```python
from build123d import *

# Parameters (mm, degrees)
BASPROSKE_W        = 12.7
BASPROSKE_H        = 33
TOOTHCUT_DEPTH     = 49.366207211
TEETHCUTS_COUNT    = 20
TEETHCUTS_ANGLE    = 342
BORSKE_R           = 5
BORE_DEPTH         = 50.0000508
CUT_EXTRUDE1_START = -6.35
CUT_EXTRUDE1_DEPTH = 6.35


with BuildPart() as part:
    # BasProSke → Base-Revolve (revolve)
    with BuildSketch(Plane(origin=(0, 0, 0), x_dir=(1, 0, 0), z_dir=(0, 1, 0)), mode=Mode.PRIVATE) as base_revolve_sk:
        with Locations((6.35, 16.5)):
            Rectangle(BASPROSKE_W, BASPROSKE_H)
    revolve(base_revolve_sk.sketch.rotate(Axis((-10, 0, 0), (1, 0, 0)), 180), axis=Axis((-10, 0, 0), (1, 0, 0)))

    # TooCutSke → ToothCut (cut, through all)
    with BuildSketch(Plane(origin=(0, 0, 0), x_dir=(0, 0, -1), z_dir=(1, 0, 0))):
        with BuildLine():
            ThreePointArc((1.489278925, 26.206717637), (0, 26.249), (-1.489278925, 26.206717637))
            ThreePointArc((-1.489278925, 26.206717637), (-2.448651415, 29.690511169), (-4.401620335, 32.730762038))
            ThreePointArc((-4.401620335, 32.730762038), (0, 33.0254), (4.401620335, 32.730762038))
            ThreePointArc((4.401620335, 32.730762038), (2.448651415, 29.690511169), (1.489278925, 26.206717637))
        make_face()
    toothcut = extrude(amount=TOOTHCUT_DEPTH, mode=Mode.SUBTRACT)

    # TeethCuts: ToothCut ×20 about axis
    teethcuts_axis = Axis((-10, 0, 0), (1, 0, 0))
    for i in range(1, TEETHCUTS_COUNT):
        add(toothcut.rotate(teethcuts_axis, i * TEETHCUTS_ANGLE / (TEETHCUTS_COUNT - 1)), mode=Mode.SUBTRACT)

    # BorSke → Bore (cut, symmetric)
    with BuildSketch(Plane(origin=(0, 0, 0), x_dir=(0, 0, -1), z_dir=(1, 0, 0))):
        with Locations(Location((0, 0, 0), (0, 0, 180))):
            Circle(BORSKE_R)
    extrude(amount=BORE_DEPTH, both=True, mode=Mode.SUBTRACT)

    # Sketch1 → Cut-Extrude1 (cut)
    with BuildSketch(Plane(origin=(12.7, 0, 0), x_dir=(0, 0, -1), z_dir=(1, 0, 0)).offset(CUT_EXTRUDE1_START)):
        with BuildLine():
            ThreePointArc((-32.707837592, 4.381479207), (-29.676574647, 2.442440757), (-26.206717637, 1.489278925))
            ThreePointArc((-26.206717637, 1.489278925), (-26.249, 0), (-26.206717637, -1.489278925))
            ThreePointArc((-26.206717637, -1.489278925), (-29.676574647, -2.442440757), (-32.707837592, -4.381479207))
            ThreePointArc((-32.707837592, -4.381479207), (-32.59371524, -5.162337346), (-32.460953611, -5.940243315))
            ThreePointArc((-32.460953611, -5.940243315), (-28.978855401, -6.847666703), (-25.384282076, -6.68193269))
            ThreePointArc((-25.384282076, -6.68193269), (-24.964282496, -8.111387085), (-24.463857082, -9.514709543))
            ThreePointArc((-24.463857082, -9.514709543), (-27.469343998, -11.493465099), (-29.753050541, -14.274312016))
            ThreePointArc((-29.753050541, -14.274312016), (-29.403215298, -14.981686491), (-29.036565322, -15.680493433))
            ThreePointArc((-29.036565322, -15.680493433), (-25.444483881, -15.467476836), (-22.077056123, -14.199070178))
            ThreePointArc((-22.077056123, -14.199070178), (-21.235887085, -15.428775087), (-20.326303746, -16.608774097))
            ThreePointArc((-20.326303746, -16.608774097), (-22.573222567, -19.419428996), (-23.885827601, -22.76987571))
            ThreePointArc((-23.885827601, -22.76987571), (-23.334523779, -23.334523779), (-22.76987571, -23.885827601))
            ThreePointArc((-22.76987571, -23.885827601), (-19.419428996, -22.573222567), (-16.608774097, -20.326303746))
            ThreePointArc((-16.608774097, -20.326303746), (-15.428775087, -21.235887085), (-14.199070178, -22.077056123))
            ThreePointArc((-14.199070178, -22.077056123), (-15.467476836, -25.444483881), (-15.680493433, -29.036565322))
            ThreePointArc((-15.680493433, -29.036565322), (-14.981686491, -29.403215298), (-14.274312016, -29.753050541))
            ThreePointArc((-14.274312016, -29.753050541), (-11.493465099, -27.469343998), (-9.514709543, -24.463857082))
            ThreePointArc((-9.514709543, -24.463857082), (-8.111387085, -24.964282496), (-6.68193269, -25.384282076))
            ThreePointArc((-6.68193269, -25.384282076), (-6.847666703, -28.978855401), (-5.940243315, -32.460953611))
            ThreePointArc((-5.940243315, -32.460953611), (-5.162337346, -32.59371524), (-4.381479207, -32.707837592))
            ThreePointArc((-4.381479207, -32.707837592), (-2.442440757, -29.676574647), (-1.489278925, -26.206717637))
            ThreePointArc((-1.489278925, -26.206717637), (0, -26.249), (1.489278925, -26.206717637))
            ThreePointArc((1.489278925, -26.206717637), (2.442440757, -29.676574647), (4.381479207, -32.707837592))
            ThreePointArc((4.381479207, -32.707837592), (5.162337346, -32.59371524), (5.940243315, -32.460953611))
            ThreePointArc((5.940243315, -32.460953611), (6.847666703, -28.978855401), (6.68193269, -25.384282076))
            ThreePointArc((6.68193269, -25.384282076), (8.111387085, -24.964282496), (9.514709543, -24.463857082))
            ThreePointArc((9.514709543, -24.463857082), (11.493465099, -27.469343998), (14.274312016, -29.753050541))
            ThreePointArc((14.274312016, -29.753050541), (14.981686491, -29.403215298), (15.680493433, -29.036565322))
            ThreePointArc((15.680493433, -29.036565322), (15.467476836, -25.444483881), (14.199070178, -22.077056123))
            ThreePointArc((14.199070178, -22.077056123), (15.428775087, -21.235887085), (16.608774097, -20.326303746))
            ThreePointArc((16.608774097, -20.326303746), (19.419428996, -22.573222567), (22.76987571, -23.885827601))
            ThreePointArc((22.76987571, -23.885827601), (23.334523779, -23.334523779), (23.885827601, -22.76987571))
            ThreePointArc((23.885827601, -22.76987571), (22.573222567, -19.419428996), (20.326303746, -16.608774097))
            ThreePointArc((20.326303746, -16.608774097), (21.235887085, -15.428775087), (22.077056123, -14.199070178))
            ThreePointArc((22.077056123, -14.199070178), (25.444483881, -15.467476836), (29.036565322, -15.680493433))
            ThreePointArc((29.036565322, -15.680493433), (29.403215298, -14.981686491), (29.753050541, -14.274312016))
            ThreePointArc((29.753050541, -14.274312016), (27.469343998, -11.493465099), (24.463857082, -9.514709543))
            ThreePointArc((24.463857082, -9.514709543), (24.964282496, -8.111387085), (25.384282076, -6.68193269))
            ThreePointArc((25.384282076, -6.68193269), (28.978855401, -6.847666703), (32.460953611, -5.940243315))
            ThreePointArc((32.460953611, -5.940243315), (32.59371524, -5.162337346), (32.707837592, -4.381479207))
            ThreePointArc((32.707837592, -4.381479207), (29.676574647, -2.442440757), (26.206717637, -1.489278925))
            ThreePointArc((26.206717637, -1.489278925), (26.249, 0), (26.206717637, 1.489278925))
            ThreePointArc((26.206717637, 1.489278925), (29.676574647, 2.442440757), (32.707837592, 4.381479207))
            ThreePointArc((32.707837592, 4.381479207), (32.59371524, 5.162337346), (32.460953611, 5.940243315))
            ThreePointArc((32.460953611, 5.940243315), (28.978855401, 6.847666703), (25.384282076, 6.68193269))
            ThreePointArc((25.384282076, 6.68193269), (24.964282496, 8.111387085), (24.463857082, 9.514709543))
            ThreePointArc((24.463857082, 9.514709543), (27.469343998, 11.493465099), (29.753050541, 14.274312016))
            ThreePointArc((29.753050541, 14.274312016), (29.403215298, 14.981686491), (29.036565322, 15.680493433))
            ThreePointArc((29.036565322, 15.680493433), (25.444483881, 15.467476836), (22.077056123, 14.199070178))
            ThreePointArc((22.077056123, 14.199070178), (21.235887085, 15.428775087), (20.326303746, 16.608774097))
            ThreePointArc((20.326303746, 16.608774097), (22.573222567, 19.419428996), (23.885827601, 22.76987571))
            ThreePointArc((23.885827601, 22.76987571), (23.334523779, 23.334523779), (22.76987571, 23.885827601))
            ThreePointArc((22.76987571, 23.885827601), (19.419428996, 22.573222567), (16.608774097, 20.326303746))
            ThreePointArc((16.608774097, 20.326303746), (15.428775087, 21.235887085), (14.199070178, 22.077056123))
            ThreePointArc((14.199070178, 22.077056123), (15.467476836, 25.444483881), (15.680493433, 29.036565322))
            ThreePointArc((15.680493433, 29.036565322), (14.981686491, 29.403215298), (14.274312016, 29.753050541))
            ThreePointArc((14.274312016, 29.753050541), (11.493465099, 27.469343998), (9.514709543, 24.463857082))
            ThreePointArc((9.514709543, 24.463857082), (8.111387085, 24.964282496), (6.68193269, 25.384282076))
            ThreePointArc((6.68193269, 25.384282076), (6.847666703, 28.978855401), (5.940243315, 32.460953611))
            ThreePointArc((5.940243315, 32.460953611), (5.162337346, 32.59371524), (4.381479207, 32.707837592))
            ThreePointArc((4.381479207, 32.707837592), (2.442440757, 29.676574647), (1.489278925, 26.206717637))
            ThreePointArc((1.489278925, 26.206717637), (0, 26.249), (-1.489278925, 26.206717637))
            ThreePointArc((-1.489278925, 26.206717637), (-2.442440757, 29.676574647), (-4.381479207, 32.707837592))
            ThreePointArc((-4.381479207, 32.707837592), (-5.162337346, 32.59371524), (-5.940243315, 32.460953611))
            ThreePointArc((-5.940243315, 32.460953611), (-6.847666703, 28.978855401), (-6.68193269, 25.384282076))
            ThreePointArc((-6.68193269, 25.384282076), (-8.111387085, 24.964282496), (-9.514709543, 24.463857082))
            ThreePointArc((-9.514709543, 24.463857082), (-11.493465099, 27.469343998), (-14.274312016, 29.753050541))
            ThreePointArc((-14.274312016, 29.753050541), (-14.981686491, 29.403215298), (-15.680493433, 29.036565322))
            ThreePointArc((-15.680493433, 29.036565322), (-15.467476836, 25.444483881), (-14.199070178, 22.077056123))
            ThreePointArc((-14.199070178, 22.077056123), (-15.428775087, 21.235887085), (-16.608774097, 20.326303746))
            ThreePointArc((-16.608774097, 20.326303746), (-19.419428996, 22.573222567), (-22.76987571, 23.885827601))
            ThreePointArc((-22.76987571, 23.885827601), (-23.334523779, 23.334523779), (-23.885827601, 22.76987571))
            ThreePointArc((-23.885827601, 22.76987571), (-22.573222567, 19.419428996), (-20.326303746, 16.608774097))
            ThreePointArc((-20.326303746, 16.608774097), (-21.235887085, 15.428775087), (-22.077056123, 14.199070178))
            ThreePointArc((-22.077056123, 14.199070178), (-25.444483881, 15.467476836), (-29.036565322, 15.680493433))
            ThreePointArc((-29.036565322, 15.680493433), (-29.403215298, 14.981686491), (-29.753050541, 14.274312016))
            ThreePointArc((-29.753050541, 14.274312016), (-27.469343998, 11.493465099), (-24.463857082, 9.514709543))
            ThreePointArc((-24.463857082, 9.514709543), (-24.964282496, 8.111387085), (-25.384282076, 6.68193269))
            ThreePointArc((-25.384282076, 6.68193269), (-28.978855401, 6.847666703), (-32.460953611, 5.940243315))
            ThreePointArc((-32.460953611, 5.940243315), (-32.59371524, 5.162337346), (-32.707837592, 4.381479207))
        make_face()
    extrude(amount=CUT_EXTRUDE1_DEPTH, mode=Mode.SUBTRACT)


solid = part.part
```
Geometry check sheet. Reference: the model listing, model coordinates, mm. A direction names the side the tool comes from. Coordinates: 2 decimals unless noted, no trailing zeros. Loops run counter-clockwise (first coordinate to the right, second up) from the corner with the lowest first, then second, coordinate; pieces in that order, holes last. Notation, with made-up numbers: (29.5, 6.5) -> (78.5, 6.5) arc R20 cw to (78.5, 18.5) -> close; hole circle Ø3 at (40.5, 46.5). An arc over 180 degrees is marked (long way). Put each result on its own line as item: value.
1) Cross-section at C-C on z = 27. Record the boundary of the cut face in (x, y).
Result set:
outline: (0, -15.69) -> (6.35, -15.69) -> (6.35, -11.09) -> (0, -11.09) -> close; (0, -6.89) -> (6.35, -6.89) -> (6.35, -1.61) -> (0, -1.61) -> close; (0, 1.61) -> (6.35, 1.61) -> (6.35, 6.89) -> (0, 6.89) -> close; (0, 11.09) -> (6.35, 11.09) -> (6.35, 15.69) -> (0, 15.69) -> close
2) Tool access check on faces 1 (the cylindrical face through (3.131, -6.853, -28.929)), 2 (the cylindrical face through (3.13, 19.38, -22.55)), 3 (the cylindrical face through (3.13, -2.42, 29.63)). Record the directions out of +Z, -Z, +X, -X, +Y, -Y that give a thin tool (end or side, any length) a straight path to the whole face; none if there is none.
Result set:
face 1: +X, -X
face 2: -Z, +X, -X
face 3: +Z, +X, -X
3) Cross-section at D-D on y = -27.5. Record the boundary of the cut face in (x, z).
Result set:
outline: (0, -15.72) -> (6.35, -15.72) -> (6.35, -11.52) -> (0, -11.52) -> close; (0, -6.91) -> (6.35, -6.91) -> (6.35, -1.71) -> (0, -1.71) -> close; (0, 1.71) -> (6.35, 1.71) -> (6.35, 6.91) -> (0, 6.91) -> close; (0, 11.52) -> (6.35, 11.52) -> (6.35, 15.72) -> (0, 15.72) -> close
4) Gauge pin test, flat ends, axial feed: pin 1 Ø6 at (y, z) = (0, 0) entering from -X; pin 2 Ø1 at (x, y) = (1, 12) entering from -Z; pin 3 Ø2 at (x, z) = (5.5, 17.5) entering from +Y; pin 4 Ø1 at (x, y) = (4.5, 13.5) entering from +Z. Record the tip position at first contact, or that the pin passes through.
Result set:
pin 1: passes through
pin 2: stops at z = -28.46
pin 3: stops at y = 21.98
pin 4: stops at z = 29.58
5) Release check for a two-part mould opening along Y. For faces 4 (the cylindrical face through (3.131, -29.029, -6.842)), 5 (the cylindrical face through (3.219, 5.173, 32.592)), 6 (the cylindrical face through (3.219, -5.151, 32.595)) record: released by +Y, released by -Y, zero draft, split by the parting line, or undercut.
Result set:
face 4: undercut
face 5: released by +Y
face 6: released by -Y
6) Thickness scan on line 1 (Z direction, x = 3.25, y = 27); line 2 (Y direction, x = 4.5, z = 23). Record the ranges inside material, lowest first.
Result set:
line 1: z = -15.69 to -11.09, -6.89 to -1.61, 1.61 to 6.89, 11.09 to 15.69
line 2: y = -23.66 to -20.23, -14.67 to 14.67, 20.23 to 23.66
7) Cross-section at A-A on y = 0. Record the boundary of the cut face in (x, z).
Result set:
outline: (0, -26.25) -> (6.35, -26.25) -> (6.35, -5) -> (0, -5) -> close; (0, 5) -> (6.35, 5) -> (6.35, 26.25) -> (0, 26.25) -> close
